Here's how the part is built. I have some questions about the finished solid (model axes, mm). Face numbers are marked on the shaded views. A direction names the side the tool comes from. Coordinates: 2 decimals unless noted, no trailing zeros. Order: outer loops, then holes, each group sorted by start corner. A loop starts at its lowest first (then second) coordinate and runs counter-clockwise, first axis right, second up. Notation, with made-up numbers: (-40, 14) - (-8, 14) arc R30 ccw to (-8, 53) - close; hole circle Ø10 at (78, 82). An arc over 180 degrees is marked (long way). Use one line per item in the form item = value. Start each with the question number.
from build123d import *

# Parameters (mm, degrees)
CHAMFER_1_SIZE              = 1.5
CHAMFER_1_SIZE2             = 0.264490471
CHAMFER_2_SIZE              = 1
SKETCH_2_W                  = 1.6
SKETCH_2_H                  = 2.408745076
SKETCH_6_R                  = 10
EXTRUDE_2_DEPTH             = 42.4
EXTRUDE_2_DIRECTION_2_REACH = 111.159
CHAMFER_5_SIZE              = 1.5
CHAMFER_5_SIZE2             = 0.264490471
CUT_EXTRUDE_2_DEPTH         = 3.5
CHAMFER_6_SIZE              = 1.5
EXTRUDE_START               = -15.5
SKETCH_9_R                  = 14.5
SKETCH_9_R_2                = 13
EXTRUDE_3_DEPTH             = 15.5
CHAMFER_7_SIZE              = 1.5
FILLET_1_R                  = 0.4


with BuildPart() as part:
    # Эскиз1 → Повернуть1 (revolve)
    with BuildSketch(Plane.XY, mode=Mode.PRIVATE) as revolve_1_sk:
        Polygon((0, 0), (0, 13), (30, 13), (30, 10), (51, 10), (51, 9), (55, 9), (55, 0), align=None)
    revolve(revolve_1_sk.sketch.rotate(Axis((0, 0, 0), (1, 0, 0)), 90), axis=Axis((0, 0, 0), (1, 0, 0)))

    # Зеркальное отражение1: part across plane


with BuildPart() as part_1:
    add(part.part)
    add(part.part.mirror(Plane(origin=(0, 0, 0), x_dir=(0, 0, 1), z_dir=(1, 0, 0))))

    # Фаска1
    chamfer_1_edges = [part_1.edges().sort_by_distance(p)[0] for p in [
        (51, 0, -10),
    ]]
    chamfer_1_side = [part_1.faces().sort_by_distance(p)[0] for p in [
        (40.5, 0, -10),
    ]]
    chamfer(chamfer_1_edges, length=CHAMFER_1_SIZE, length2=CHAMFER_1_SIZE2, reference=chamfer_1_side[0])

    # Фаска2
    chamfer_2_edges = [part_1.edges().sort_by_distance(p)[0] for p in [
        (55, 0, -9),
    ]]
    chamfer(chamfer_2_edges, length=CHAMFER_2_SIZE)

    # Эскиз2 → Вырез-Повернуть1 (revolve, cut)
    with BuildSketch(Plane(origin=(0, 0, 0), x_dir=(1, 0, 0), z_dir=(0, 1, 0)), mode=Mode.PRIVATE) as cut_revolve_1_sk:
        with Locations((51.8, 9.704372538)):
            Rectangle(SKETCH_2_W, SKETCH_2_H)
    cut_revolve_1 = revolve(cut_revolve_1_sk.sketch.rotate(Axis((0, 0, 0), (1, 0, 0)), 180), axis=Axis((0, 0, 0), (1, 0, 0)), mode=Mode.SUBTRACT)

    # Зеркальное отражение2: Вырез-Повернуть1 across plane
    add(cut_revolve_1.mirror(Plane(origin=(0, 0, 0), x_dir=(0, 0, 1), z_dir=(1, 0, 0))), mode=Mode.SUBTRACT)

    # Эскиз6 → Бобышка-Вытянуть2 (add)
    with BuildSketch(Plane(origin=(-52.6, 0, 0), x_dir=(0, 0, -1), z_dir=(1, 0, 0))):
        with Locations(Location((0, 0, 0), (0, 0, 180))):
            Circle(SKETCH_6_R)
    extrude(amount=-EXTRUDE_2_DEPTH)

    # Эскиз6 → Бобышка-Вытянуть2 direction 2 (add, up to next)
    with BuildSketch(Plane(origin=(-52.6, 0, 0), x_dir=(0, 0, -1), z_dir=(1, 0, 0)), mode=Mode.PRIVATE) as extrude_2_direction_2_sk1:
        with Locations(Location((0, 0, 0), (0, 0, 180))):
            Circle(SKETCH_6_R)
    extrude_2_direction_2_tool1 = extrude(extrude_2_direction_2_sk1.sketch, amount=EXTRUDE_2_DIRECTION_2_REACH, mode=Mode.PRIVATE) - part_1.part
    add(extrude_2_direction_2_tool1.solids().sort_by_distance((-52.6, 0, 0))[0])

    # Фаска5
    chamfer_5_edges = [part_1.edges().sort_by_distance(p)[0] for p in [
        (-95, 0, -10),
    ]]
    chamfer_5_side = [part_1.faces().sort_by_distance(p)[0] for p in [
        (-73.8, 0, -10),
    ]]
    chamfer(chamfer_5_edges, length=CHAMFER_5_SIZE, length2=CHAMFER_5_SIZE2, reference=chamfer_5_side[0])

    # Зеркальное отражение5: Вырез-Повернуть1 across plane
    add(cut_revolve_1.mirror(Plane(origin=(-20, 0, 0), x_dir=(0, 0, 1), z_dir=(1, 0, 0))), mode=Mode.SUBTRACT)

    # Эскиз8 → Вырез-Вытянуть2 (cut)
    with BuildSketch(Plane.XY.offset(10)):
        with BuildLine():
            Line((-119, 3), (-71, 3))
            ThreePointArc((-71, 3), (-68, 0), (-71, -3))
            Line((-71, -3), (-119, -3))
            ThreePointArc((-119, -3), (-122, 0), (-119, 3))
        make_face()
    extrude(amount=-CUT_EXTRUDE_2_DEPTH, mode=Mode.SUBTRACT)

    # Фаска6
    chamfer_6_edges = [part_1.edges().sort_by_distance(p)[0] for p in [
        (-30, 0, -13),
    ]]
    chamfer(chamfer_6_edges, length=CHAMFER_6_SIZE)

    # Эскиз9 → Бобышка-Вытянуть3 (add)
    with BuildSketch(Plane(origin=(30, 0, 0), x_dir=(0, 0, -1), z_dir=(1, 0, 0)).offset(EXTRUDE_START)):
        Circle(SKETCH_9_R)
        Circle(SKETCH_9_R_2, mode=Mode.SUBTRACT)
    extrude(amount=EXTRUDE_3_DEPTH)

    # Фаска7
    chamfer_7_edges = [part_1.edges().sort_by_distance(p)[0] for p in [
        (30, 0, 14.5),
    ]]
    chamfer(chamfer_7_edges, length=CHAMFER_7_SIZE)

    # Скругление1
    fillet_1_edges = [part_1.edges().sort_by_distance(p)[0] for p in [
        (-68, 0, 6.5),
        (-83, 3, 6.5),
        (-83, -3, 6.5),
    ]]
    fillet(fillet_1_edges, radius=FILLET_1_R)


solid = part_1.part
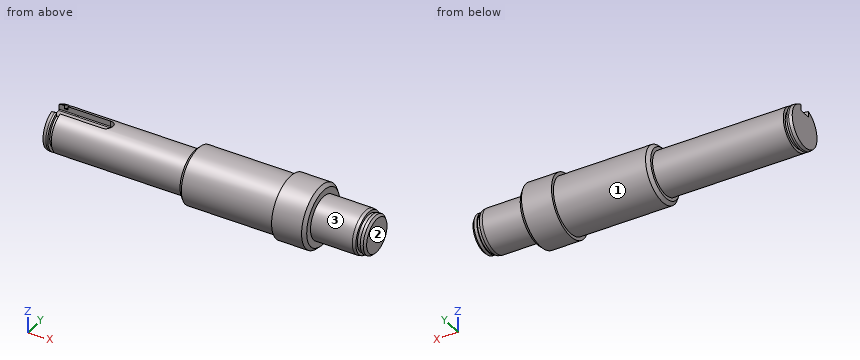
1) Which directions (+Z, -Z, +X, -X, +Y, -Y) give clear straight access to the entire face, cutting with the end or side of a thin tool? Please do the marked faces 1, 2 and 3.
2) For pin 1 (4 mm diameter, centred on x = -2.5, z = -5, fed in from -Y); pin 2 (8 mm diameter, centred on x = -54, y = 0.5, fed in from +Z); pin 3 (12 mm diameter, centred on y = 10.5, z = -2, fed in from -X); pin 4 (8 mm diameter, centred on x = -75.5, z = 10, fed in from -Y), each with a flat end and sliding along its axis, tell me the tip position at first contact or that it passes through.
3) Suppose I cut it at A-A, the plane x = 9.5. List the corners of the cut face in (y, z) for me, then the cut area to 3 significant figures.
4) I need wall thicknesses on probe 1 along X at (y, z) = (8.75, -6.75); probe 2 along X at (y, z) = (7.75, -4.5); probe 3 along Y at (x, z) = (-73, 5.25). Which ranges of each line are inside material? Lowest first, please. Write a range as [from, to].
From the geometry:
q1.face_1 = -X
q1.face_2 = +Z, -Z, +X, +Y, -Y
q1.face_3 = +X
q2.pin_1 = -12.65
q2.pin_2 = 10
q2.pin_3 = -95
q2.pin_4 = -8
q3.outline = circle Ø26 at (0, 0)
q3.area = 531 mm2
q4.probe_1 = [-30, 30]
q4.probe_2 = [-95, -92.6], [-91, 51], [52.6, 54.04]
q4.probe_3 = [-8.51, 8.51]
